Answer from the drawing. Dimensions are ordinates in mm from the lowest x, y and z of the part. Round coordinates to 2 decimals unless told otherwise and drop trailing zeros. Loops run counter-clockwise (first coordinate to the right, second up) from the corner with the lowest first, then second, coordinate; pieces in that order, holes last.
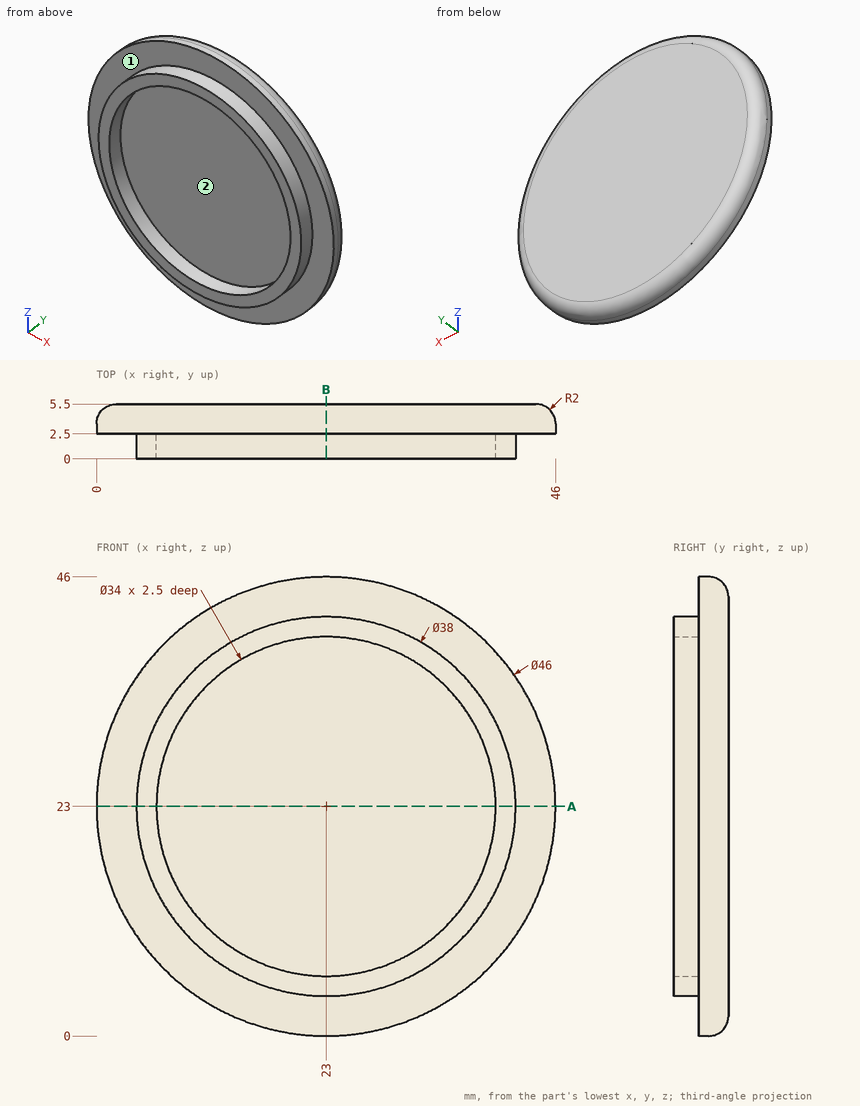
1. Find section A-A (z = 23). Write down the section's boundary in (x, y).
Answer key:
outline: (0, 2.5) - (4, 2.5) - (4, 0) - (6, 0) - (6, 2.5) - (40, 2.5) - (40, 0) - (42, 0) - (42, 2.5) - (46, 2.5) - (46, 3.5) arc R2 ccw to (44, 5.5) - (2, 5.5) arc R2 ccw to (0, 3.5) - close
2. Find section B-B (x = 23). Write down the section's boundary in (y, z).
Answer key:
outline: (0, 4) - (2.5, 4) - (2.5, 0) - (3.5, 0) arc R2 ccw to (5.5, 2) - (5.5, 44) arc R2 ccw to (3.5, 46) - (2.5, 46) - (2.5, 42) - (0, 42) - (0, 40) - (2.5, 40) - (2.5, 6) - (0, 6) - close
3. Given pin 1 (23 mm diameter, centred on x = 12.5, z = 20, fed in from -Y); pin 2 (10 mm diameter, centred on x = 21.5, z = 30.5, fed in from -Y); pin 3 (2 mm diameter, centred on x = 28.5, y = 3, fed in from -Z); pin 4 (2 mm diameter, centred on x = 26, y = 2.5, fed in from -Z), each flat-ended and moving along its own axis, determine where each tip first touches the part or whether it passes through.
Answer key:
pin 1: stops at y = 0
pin 2: stops at y = 2.5
pin 3: stops at z = 0.44
pin 4: stops at z = 0.09
4. Determine the mould class of the marked faces 1 and 2 for opening direction X: +X half, -X half, draft (parallel to the pull), parting line (faces both ways), or undercut.
Answer key:
face 1: draft
face 2: undercut
5. Consider probe 1 along X at (y, z) = (1.9, 23); probe 2 along Y at (x, z) = (10, 29); probe 3 along X at (y, z) = (2.4, 38). Determine where each line is inside the solid, lowest interval first.
Answer key:
probe 1: x = 4 to 6, 40 to 42
probe 2: y = 2.5 to 5.5
probe 3: x = 11.34 to 15, 31 to 34.66
